Drawing for the job (mm, zero at the part's lowest x, y, z). Give positions to 0.01 mm unless a question says otherwise; leave off trailing zeros. Order: outer loops, then holes, each group sorted by start corner. A loop starts at its lowest first (then second) coordinate and runs counter-clockwise, first axis right, second up. Notation, with made-up numbers: (-1, 59.25) - (28, 59.25) arc R24 cw to (28, 71.25) - close; hole circle Ø7 at (81.5, 88.25). An arc over 180 degrees is marked (long way). Use a Markdown table: item, result. Add a question column.
(1) Flat gauge pins, fed straight in: pin 1 (3 mm diameter, centred on x = 2.5, y = 27, fed in from -Z); pin 2 (1.8 mm diameter, centred on x = 2.5, z = 6, fed in from +Y); pin 3 (2 mm diameter, centred on x = 3.5, z = 95, fed in from +Y). Where does each tip first touch, or does it go through?
(2) Wall check: line 1 (Z direction, x = 3.4, y = 17); line 2 (Z direction, x = 1.3, y = 37); line 3 (Y direction, x = 1.85, z = 115.5). Give the ranges that are in metal, low to high.
(3) Slice it at B-B (z = 109.5). Write the cut outline in (x, y), then the cut area to 3 significant figures.
(4) Slice it at A-A (x = 2.45). Write the cut outline in (y, z).
(5) Slice it at C-C (y = 26). Write the cut outline in (x, z), then the cut area to 3 significant figures.
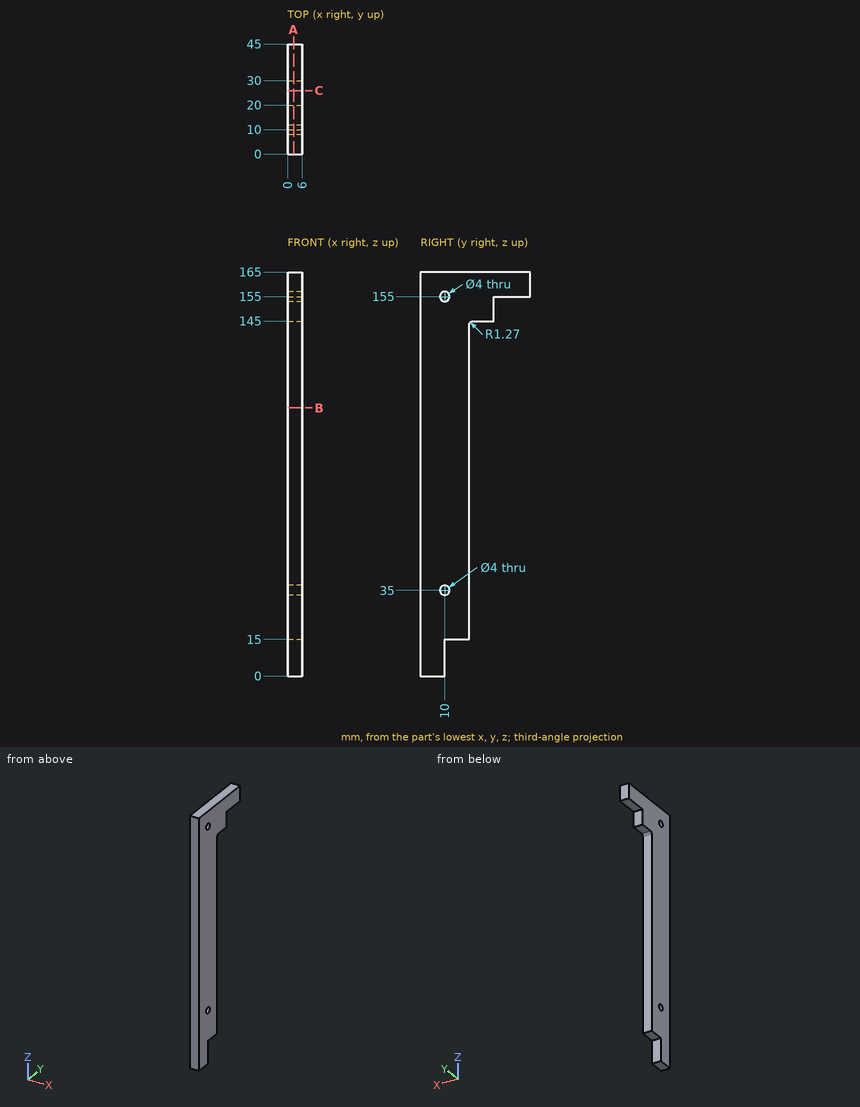
Solution:
| question | item | result |
|---|---|---|
| 1 | pin 1 | z = 145 |
| 1 | pin 2 | y = 10 |
| 1 | pin 3 | y = 20 |
| 2 | line 1 | 15 to 165 |
| 2 | line 2 | 155 to 165 |
| 2 | line 3 | 0 to 20 |
| 3 | outline | (0, 0) - (6, 0) - (6, 20) - (0, 20) - close |
| 3 | area | 120 mm2 |
| 4 | outline | (0, 0) - (10, 0) - (10, 15) - (20, 15) - (20, 143.73) arc R1.27 cw to (21.27, 145) - (30, 145) - (30, 155) - (45, 155) - (45, 165) - (0, 165) - close; hole circle Ø4 at (10, 35); hole circle Ø4 at (10, 155) |
| 5 | outline | (0, 145) - (6, 145) - (6, 165) - (0, 165) - close |
| 5 | area | 120 mm2 |
